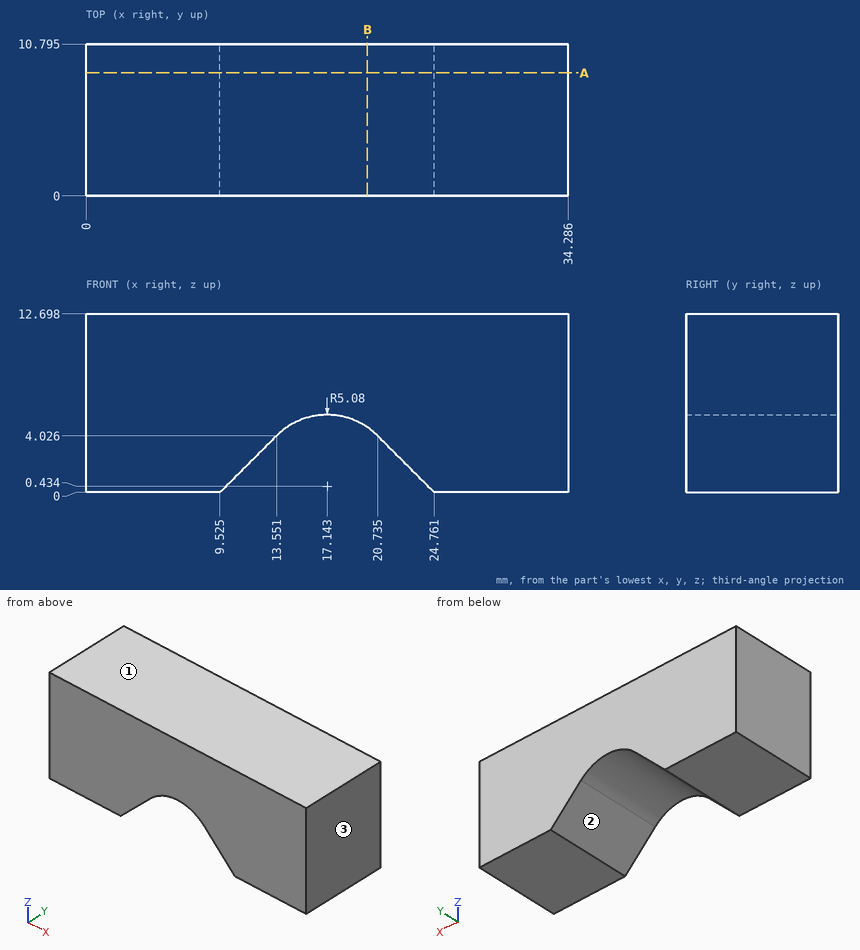
Geometry check sheet. Reference: drawing and pictorial views, mm from the part's lowest x, y, z. Give positions to 0.01 mm unless a question says otherwise; leave off trailing zeros. Write each loop counter-clockwise with the first axis right and the second up, starting at its lowest first coordinate (ties: lowest second). Pieces come first, ordered by that corner, then holes.
Item 1: Gauge pin test, flat ends, axial feed: pin 1 (1.5 mm diameter, centred on x = 21.5, y = 7.5, fed in from -Z); pin 2 (4 mm diameter, centred on x = 17, y = 6.5, fed in from -Z). Record the tip position at first contact, or that the pin passes through.
Item 2: Cross-section at A-A (y = 8.75). Enter the section's corners in (x, z) (1 decimal), and give its area (3 significant figures).
Item 3: Draft check along X on the marked faces 1, 2 and 3. Enter one of: released by +X, released by -X, zero draft, split by the parting line, or undercut.
Item 4: Scan lines: L1, parallel to X at y = 6.75, z = 2.75 (1 decimal); L2, parallel to X at y = 7, z = 1.5 (1 decimal); L3, parallel to Z at x = 11.5, y = 4.75 (1 decimal). Record each from-to range of solid material in increasing order.
Item 5: Cross-section at B-B (x = 20). Enter the section's corners in (y, z) (1 decimal).
Report:
1. pin 1: stops at z = 2.51
1. pin 2: stops at z = 5.04
2. outline: (0, 0) - (9.5, 0) - (13.6, 4) arc R5.1 cw to (20.7, 4) - (24.8, 0) - (34.3, 0) - (34.3, 12.7) - (0, 12.7) - close
2. area: 383 mm2
3. face 1: zero draft
3. face 2: undercut
3. face 3: released by +X
4. L1: x = 0 to 12.3, 22 to 34.3
4. L2: x = 0 to 11, 23.3 to 34.3
4. L3: z = 2 to 12.7
5. outline: (0, 4.6) - (10.8, 4.6) - (10.8, 12.7) - (0, 12.7) - close
